Check sheet for the modelled part. Datum: model origin and axes. Units: mm. A direction names the side the tool comes from. Coordinates: 2 decimals unless noted, no trailing zeros.
```python
from build123d import *

# Parameters (mm, degrees)
F0_W     = 31.75
F0_H     = 57.15
F1_DEPTH = 406.4
F4_D     = 7.9375
F4_DEPTH = 20.6883
F4_TIP   = 2.3846655818
F5_D     = 3.7973
F5_DEPTH = 19.0881
F5_TIP   = 1.1408240143


with BuildPart() as f1:
    # F0 (on Front) → F1 (new body)
    with BuildSketch(Plane.XZ):
        with Locations((15.875, 28.575)):
            Rectangle(F0_W, F0_H)
    extrude(amount=F1_DEPTH)

    # F4
    with Locations(Plane.XY.offset(57.15)):
        with Locations((15.875, -381), (15.875, -203.2), (15.875, -25.4)):
            Hole(F4_D / 2, depth=F4_DEPTH)
            with Locations((0, 0, -(F4_DEPTH + F4_TIP / 2))):  # 118° drill point
                Cone(0, F4_D / 2, F4_TIP, mode=Mode.SUBTRACT)

    # F5
    with Locations(Plane.YZ.offset(31.75)):
        with Locations((-374.65, 25.4), (-146.05, 25.4), (-31.75, 25.4), (-260.35, 25.4)):
            Hole(F5_D / 2, depth=F5_DEPTH)
            with Locations((0, 0, -(F5_DEPTH + F5_TIP / 2))):  # 118° drill point
                Cone(0, F5_D / 2, F5_TIP, mode=Mode.SUBTRACT)


solid = f1.part
```
1) Set-up check for faces 1 (the cylindrical face through (12.2, -26.9, 46.7)), 2 (the flat face through (16, -200, 0)): record each of +Z, -Z, +X, -X, +Y, -Y from which the full face is reachable in a straight line by a thin tool's end or side.
Answer sheet:
face 1: +Z
face 2: -Z, +X, -X, +Y, -Y
2) Mould release check, pull along Y, two halves, no side actions. Record for faces 3 (the flat face through (16, 0, 29)), 4 (the cylindrical face through (16.392, -377.065, 46.661)), 5 (the flat face through (0, -200, 28)): +Y half, -Y half, draft (parallel to the pull), parting line (faces both ways), or undercut.
Answer sheet:
face 3: +Y half
face 4: undercut
face 5: draft
3) Scan lines: line 1 (Y direction, x = 16.5, z = 53); line 2 (X direction, y = -25, z = 49); line 3 (Z direction, x = 16.5, y = -30.5). Record each from-to range of solid material in increasing order.
Answer sheet:
line 1: y = -406.4 to -384.92, -377.08 to -207.12, -199.28 to -29.32, -21.48 to 0
line 2: x = 0 to 11.93, 19.82 to 31.75
line 3: z = 0 to 23.97, 26.83 to 57.15
